Geometry: final body of the model. Coordinates: model frame, mm. Face numbers are marked on the shaded views. A direction names the side the tool comes from. Coordinates: 2 decimals unless noted, no trailing zeros. Write each loop counter-clockwise with the first axis right and the second up, starting at its lowest first coordinate (ties: lowest second). Pieces come first, ordered by that corner, then holes. Notation, with made-up numbers: (65.5, -33) - (120.5, -33) arc R22 ccw to (120.5, -9) - close; hole circle Ø10 at (-19.5, 75). An arc over 180 degrees is marked (long way). Put each result on its own line as item: value.
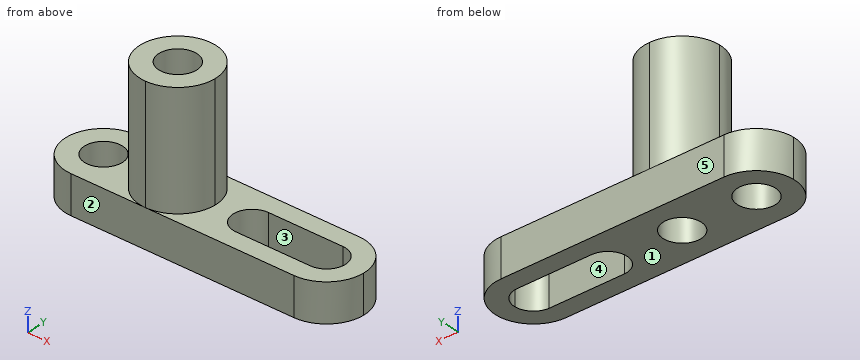
```python
from build123d import *

# Parameters (mm, degrees)
F1_DEPTH  = 25.4
F3_DEPTH  = 38.1
F4_R      = 6.35
F5_DEPTH  = 63.5
F6_R      = 6.35
F7_DEPTH  = 25.4
F9_DEPTH  = 25.4
F11_DEPTH = 25.4
F13_DEPTH = 25.4


with BuildPart() as f1:
    # F0 (on Front) → F1 (new body)
    with BuildSketch(Plane.XZ):
        Polygon((-101.6, 0), (0, 0), (0, 12.7), (-50.8, 12.7), (-50.8, 50.8), (-76.2, 50.8), (-76.2, 12.7), (-101.6, 12.7), align=None)
    extrude(amount=F1_DEPTH)

    # F2 (on face) → F3 (cut)
    with BuildSketch(Plane.XY.offset(50.8)):
        with BuildLine():
            ThreePointArc((-63.5, 0), (-54.5197438789, -3.7197438789), (-50.8, -12.7))
            Line((-50.8, -12.7), (-50.8, 0))
            Line((-50.8, 0), (-63.5, 0))
        make_face()
        with BuildLine():
            ThreePointArc((-76.2, -12.7), (-72.4802561211, -3.7197438789), (-63.5, 0))
            Line((-63.5, 0), (-76.2, 0))
            Line((-76.2, 0), (-76.2, -12.7))
        make_face()
        with BuildLine():
            Line((-76.2, -25.4), (-63.5, -25.4))
            ThreePointArc((-63.5, -25.4), (-72.4802561211, -21.6802561211), (-76.2, -12.7))
            Line((-76.2, -12.7), (-76.2, -25.4))
        make_face()
        with BuildLine():
            Line((-50.8, -25.4), (-50.8, -12.7))
            ThreePointArc((-50.8, -12.7), (-54.5197438789, -21.6802561211), (-63.5, -25.4))
            Line((-63.5, -25.4), (-50.8, -25.4))
        make_face()
    extrude(amount=-F3_DEPTH, mode=Mode.SUBTRACT)

    # F4 (on face) → F5 (cut)
    with BuildSketch(Plane.XY.offset(50.8)):
        with Locations((-63.5, -12.7)):
            Circle(F4_R)
    extrude(amount=-F5_DEPTH, mode=Mode.SUBTRACT)

    # F6 (on face) → F7 (cut)
    with BuildSketch(Plane.XY.offset(12.7)):
        with Locations((-88.9, -12.7)):
            Circle(F6_R)
    extrude(amount=-F7_DEPTH, mode=Mode.SUBTRACT)

    # F8 (on face) → F9 (cut)
    with BuildSketch(Plane.XY.offset(12.7)):
        with BuildLine():
            ThreePointArc((-101.6, -12.7), (-97.8802561211, -3.7197438789), (-88.9, 0))
            Line((-88.9, 0), (-101.6, 0))
            Line((-101.6, 0), (-101.6, -12.7))
        make_face()
        with BuildLine():
            Line((-101.6, -25.4), (-88.9, -25.4))
            ThreePointArc((-88.9, -25.4), (-97.8802561211, -21.6802561211), (-101.6, -12.7))
            Line((-101.6, -12.7), (-101.6, -25.4))
        make_face()
    extrude(amount=-F9_DEPTH, mode=Mode.SUBTRACT)

    # F10 (on face) → F11 (cut)
    with BuildSketch(Plane.XY.offset(12.7)):
        with BuildLine():
            ThreePointArc((-37.9124571555, -19.0472299219), (-33.5440480104, -17.1233247076), (-31.75, -12.7))
            ThreePointArc((-31.75, -12.7), (-33.6098719395, -8.2098719395), (-38.1, -6.35))
            ThreePointArc((-38.1, -6.35), (-44.4493074427, -12.6062183495), (-38.2875428445, -19.0472299219))
            Line((-38.2875428445, -19.0472299219), (-37.9124571555, -19.0472299219))
        make_face()
        with BuildLine():
            ThreePointArc((-38.1, -6.35), (-33.6098719395, -8.2098719395), (-31.75, -12.7))
            ThreePointArc((-31.75, -12.7), (-33.5440480104, -17.1233247076), (-37.9124571555, -19.0472299219))
            Line((-37.9124571555, -19.0472299219), (-12.8875428445, -19.0472299219))
            ThreePointArc((-12.8875428445, -19.0472299219), (-19.0493074427, -12.6062183495), (-12.7, -6.35))
            Line((-12.7, -6.35), (-38.1, -6.35))
        make_face()
        with BuildLine():
            ThreePointArc((-6.35, -12.7), (-8.2098719395, -8.2098719395), (-12.7, -6.35))
            ThreePointArc((-12.7, -6.35), (-19.0493074427, -12.6062183495), (-12.8875428445, -19.0472299219))
            Line((-12.8875428445, -19.0472299219), (-12.5124571555, -19.0472299219))
            ThreePointArc((-12.5124571555, -19.0472299219), (-8.1440480104, -17.1233247076), (-6.35, -12.7))
        make_face()
    extrude(amount=-F11_DEPTH, mode=Mode.SUBTRACT)

    # F12 (on face) → F13 (cut)
    with BuildSketch(Plane.XY.offset(12.7)):
        with BuildLine():
            ThreePointArc((-12.7, 0), (-3.7197438789, -3.7197438789), (0, -12.7))
            Line((0, -12.7), (0, 0))
            Line((0, 0), (-12.7, 0))
        make_face()
        with BuildLine():
            Line((0, -25.4), (0, -12.7))
            ThreePointArc((0, -12.7), (-3.7197438896, -21.6802561317), (-12.7000000301, -25.4))
            Line((-12.7000000301, -25.4), (0, -25.4))
        make_face()
    extrude(amount=-F13_DEPTH, mode=Mode.SUBTRACT)


solid = f1.part
```
1. Section query C-C (z = 23). Return loops of the section in (x, y), then the cut area to 3 significant figures.
Answer below:
outline: circle Ø25.4 at (-63.5, -12.7); hole circle Ø12.7 at (-63.5, -12.7)
area: 380 mm²
2. Set-up query: the marked faces 4 and 5. Return all of +Z, -Z, +X, -X, +Y, -Y with unobstructed straight access to the full face (end or side cutting, diameter ignored); none if empty.
Answer below:
face 4: +Z, -Z
face 5: +Z, -Z, +X, -X, +Y
3. Mould query, pull axis Y, two halves, no side actions, for the marked faces 1, 2 and 3. Classes: +Y half, -Y half, draft (parallel to the pull), parting line (faces both ways), or undercut.
Answer below:
face 1: draft
face 2: -Y half
face 3: undercut
4. Section query A-A (x = -35). Return loops of the section in (y, z), then the cut area to 3 significant figures.
Answer below:
outline: (-25.4, 0) - (-19.05, 0) - (-19.05, 12.7) - (-25.4, 12.7) - close; (-6.35, 0) - (0, 0) - (0, 12.7) - (-6.35, 12.7) - close
area: 161 mm²
5. Ray query, probe 1 along Y at (x, z) = (-63, 33); probe 2 along Y at (x, z) = (-32, 8); probe 3 along Z at (x, y) = (-19, -3). Return the intervals inside material, ascending. Write a range as from..to.
Answer below:
probe 1: y = -25.39..-19.03, -6.37..-0.01
probe 2: y = -25.4..-19.05, -6.35..0
probe 3: z = 0..12.7
6. Section query D-D (y = -7.75). Return loops of the section in (x, z), then the cut area to 3 significant figures.
Answer below:
outline: (-100.6, 0) - (-92.88, 0) - (-92.88, 12.7) - (-100.6, 12.7) - close; (-84.92, 0) - (-67.48, 0) - (-67.48, 50.8) - (-75.2, 50.8) - (-75.2, 12.7) - (-84.92, 12.7) - close; (-59.52, 0) - (-42.08, 0) - (-42.08, 12.7) - (-51.8, 12.7) - (-51.8, 50.8) - (-59.52, 50.8) - close; (-8.72, 0) - (-1, 0) - (-1, 12.7) - (-8.72, 12.7) - close
area: 1,230 mm²
7. Pin query (flat end, axial travel): pin 1 Ø12 at (x, z) = (-27, 22) entering from -Y; pin 2 Ø1.5 at (x, z) = (-76, 18.5) entering from +Y; pin 3 Ø4 at (x, z) = (-50.5, 41.5) entering from +Y; pin 4 Ø8 at (x, y) = (-22.5, -20.5) entering from +Z. Return the tip coordinate at first contact, or that it passes through.
Answer below:
pin 1: passes through
pin 2: stops at y = -7.88
pin 3: stops at y = -6.35
pin 4: stops at z = 12.7
8. Section query B-B (y = -14.25). Return loops of the section in (x, z), then the cut area to 3 significant figures.
Answer below:
outline: (-101.51, 0) - (-95.06, 0) - (-95.06, 12.7) - (-101.51, 12.7) - close; (-82.74, 0) - (-69.66, 0) - (-69.66, 50.8) - (-76.11, 50.8) - (-76.11, 12.7) - (-82.74, 12.7) - close; (-57.34, 0) - (-44.26, 0) - (-44.26, 12.7) - (-50.89, 12.7) - (-50.89, 50.8) - (-57.34, 50.8) - close; (-6.54, 0) - (-0.09, 0) - (-0.09, 12.7) - (-6.54, 12.7) - close
area: 987 mm²
